from build123d import *

# Parameters (mm, degrees)
F0_W     = 100
F0_H     = 75
F1_DEPTH = 2
F2_W     = 2
F2_H     = 75
F3_DEPTH = 50
F4_R     = 5
F4_R_2   = 2.75
F5_DEPTH = 100


with BuildPart() as f1:
    # F0 (on Top) → F1 (new body)
    with BuildSketch(Plane.XY):
        with Locations((-50, 37.5)):
            Rectangle(F0_W, F0_H)
    extrude(amount=F1_DEPTH)

    # F2 (on face) → F3 (join)
    with BuildSketch(Plane.XY.offset(2)):
        with Locations((-99, 37.5)):
            Rectangle(F2_W, F2_H)
        with Locations((-1, 37.5)):
            Rectangle(F2_W, F2_H)
    extrude(amount=F3_DEPTH)

    # F4 (on face) → F5 (cut)
    with BuildSketch(Plane.YZ):
        with Locations((28, 35)):
            Circle(F4_R)
        with Locations((42, 44)):
            Circle(F4_R_2)
    extrude(amount=-F5_DEPTH, mode=Mode.SUBTRACT)


solid = f1.part
Build history of the part. All positions in model axes, mm. A direction names the side the tool comes from. Round coordinates to 2 decimals unless told otherwise and drop trailing zeros. Loops run counter-clockwise (first coordinate to the right, second up) from the corner with the lowest first, then second, coordinate; pieces in that order, holes last. Notation, with made-up numbers: (-36, -19) -> (-14, -19) arc R9 cw to (-14, -7) -> close; hole circle Ø2 at (63, 19). An arc over 180 degrees is marked (long way). One line per item, written item: value. Start each with the question number.
Q1. Cut at B-B on z = 48. List the corners of the cut face in (x, y), plus the area to 3 significant figures.
Q2. Cut at A-A on y = 42. List the corners of the cut face in (x, z).
Q3. Drop flat-ended pins along their axis: pin 1 Ø25 at (y, z) = (48, 16.5) entering from +X; pin 2 Ø3 at (x, y) = (-29, 54.5) entering from +Z. Give the stop position or say it passes through.
Q4. Cut at C-C on z = 35. List the corners of the cut face in (x, y).
Q5. 3-axis set-ups, long thin cutter, end or side, ignore diameter. For faces 1 (the face through (-98, 37, 27)), 2 (the face through (-100, 37, 26)): which of +Z, -Z, +X, -X, +Y, -Y reach the whole face in a straight line?
Q6. Probe line 1 along Z through (x, y) = (-1.15, 28); line 2 along X through (y, z) = (7, 7); line 3 along Z through (x, y) = (-0.95, 42). List the from-to ranges inside material, lowest first.
Q7. Two-plate mould, pull along X, no slides. Class faces 3 (the face through (-2, 37, 27)), 4 (the face through (-51, 38, 2)), 5 (the face through (0, 37, 26)), 6 (the face through (-98.986, 39.973, 45.859)): released by +X, released by -X, zero draft, split by the parting line, or undercut.
Q8. Cut at D-D on y = 56. List the corners of the cut face in (x, z), plus the area to 3 significant figures.
Computed:
1. outline: (-100, 0) -> (-98, 0) -> (-98, 75) -> (-100, 75) -> close; (-2, 0) -> (0, 0) -> (0, 75) -> (-2, 75) -> close
1. area: 300 mm²
2. outline: (-100, 0) -> (0, 0) -> (0, 41.25) -> (-2, 41.25) -> (-2, 2) -> (-98, 2) -> (-98, 41.25) -> (-100, 41.25) -> close; (-100, 46.75) -> (-98, 46.75) -> (-98, 52) -> (-100, 52) -> close; (-2, 46.75) -> (0, 46.75) -> (0, 52) -> (-2, 52) -> close
3. pin 1: x = 0
3. pin 2: z = 2
4. outline: (-100, 0) -> (-98, 0) -> (-98, 23) -> (-100, 23) -> close; (-100, 33) -> (-98, 33) -> (-98, 75) -> (-100, 75) -> close; (-2, 0) -> (0, 0) -> (0, 23) -> (-2, 23) -> close; (-2, 33) -> (0, 33) -> (0, 75) -> (-2, 75) -> close
5. face 1: +Z, +Y, -Y
5. face 2: +Z, -Z, -X, +Y, -Y
6. line 1: 0 to 30, 40 to 52
6. line 2: -100 to -98, -2 to 0
6. line 3: 0 to 41.25, 46.75 to 52
7. face 3: undercut
7. face 4: undercut
7. face 5: released by +X
7. face 6: zero draft
8. outline: (-100, 0) -> (0, 0) -> (0, 52) -> (-2, 52) -> (-2, 2) -> (-98, 2) -> (-98, 52) -> (-100, 52) -> close
8. area: 400 mm²
